from build123d import *

# Parameters (mm, degrees)
SKETCH1_W           = 8
SKETCH1_H           = 110
BOSS_EXTRUDE1_DEPTH = 40
SKETCH2_W           = 20
SKETCH2_H           = 24
CUT_EXTRUDE1_DEPTH  = 9
FILLET1_R           = 3
SKETCH3_R           = 1.25
CUT_EXTRUDE2_DEPTH  = 41


with BuildPart() as part:
    # Sketch1 → Boss-Extrude1 (new body)
    with BuildSketch(Plane.XY):
        Rectangle(SKETCH1_W, SKETCH1_H)
    extrude(amount=-BOSS_EXTRUDE1_DEPTH)

    # Sketch2 → Cut-Extrude1 (cut, through all)
    with BuildSketch(Plane(origin=(4, 0, 0), x_dir=(0, 0, -1), z_dir=(1, 0, 0))):
        with Locations((20, 55)):
            Rectangle(SKETCH2_W, SKETCH2_H)
        with Locations((20, -55)):
            Rectangle(SKETCH2_W, SKETCH2_H)
    extrude(amount=-CUT_EXTRUDE1_DEPTH, mode=Mode.SUBTRACT)

    # Fillet1
    fillet1_edges = [part.edges().sort_by_distance(p)[0] for p in [
        (4, 55, -5),
        (-4, 55, -5),
        (-4, -55, -5),
        (4, -55, -5),
        (4, -55, -35),
        (-4, -55, -35),
        (-4, 55, -35),
        (4, 55, -35),
    ]]
    fillet(fillet1_edges, radius=FILLET1_R)

    # Sketch3 → Cut-Extrude2 (cut, through all)
    with BuildSketch(Plane.XY):
        with Locations((0, 50)):
            Circle(SKETCH3_R)
        with Locations((0, -50)):
            Circle(SKETCH3_R)
    extrude(amount=-CUT_EXTRUDE2_DEPTH, mode=Mode.SUBTRACT)


solid = part.part
Part model, mm, in its own coordinate system. A direction names the side the tool comes from. Give positions to 0.01 mm unless a question says otherwise; leave off trailing zeros. Loops run counter-clockwise (first coordinate to the right, second up) from the corner with the lowest first, then second, coordinate; pieces in that order, holes last. Notation, with made-up numbers: (-29.5, -39) -> (-1.5, -39) arc R13 cw to (-1.5, -35) -> close; hole circle Ø8 at (5.5, 36.5). An arc over 180 degrees is marked (long way). Write each question's results on one line, items separated by ' | '. Start each with the question number.
Q1. Pin check, flat tips, straight feed: P1, Ø1.5, axis at x = 0, y = -50, coming from the +Z side; P2, Ø2.5, axis at x = -0.5, z = -15, coming from the +Y side; P3, Ø4, axis at x = -1, y = 47.5, coming from the +Z side. Stop position of each tip, or through.
Q2. Band-saw the part on A-A on y = 47. List the corners of the cut face in (x, z).
Q3. Band-saw the part on C-C on z = -33. List the corners of the cut face in (x, y), plus the area to 3 significant figures.
Q4. Pull direction Y, two halves, no side cores. Call faces 1 (the face through (-0.16, -48.76, -4.93)), 2 (the face through (0, -43, -20)), 3 (the face through (-4, -1, -20)): +Y half, -Y half, draft (parallel to the pull), parting line (faces both ways), or undercut.
Q5. Which spindle directions (+Z, -Z, +X, -X, +Y, -Y) get a long thin tool onto all of the face, cutting with end or side? Do faces 4 (the face through (1, 49, -30)), 5 (the face through (1, -49, -30)), 6 (the face through (0, -55, -5)). Say none if no direction does.
Q6. Band-saw the part on D-D on y = -50. List the corners of the cut face in (x, z), plus the area to 3 significant figures.
Q7. Wall check: L1, parallel to Y at x = 0, z = -35.5; L2, parallel to Y at x = -2, z = -11; L3, parallel to Y at x = -1.5, z = -31. Give the ranges that are in metal, low to high.
Q8. Band-saw the part on B-B on x = 0. List the corners of the cut face in (y, z), plus the area to 3 significant figures.
Results are:
1) P1: passes through | P2: stops at y = 43 | P3: stops at z = 0
2) outline: (-4, -40) -> (4, -40) -> (4, -30) -> (-4, -30) -> close; (-4, -10) -> (4, -10) -> (4, 0) -> (-4, 0) -> close
3) outline: (-4, -52) arc R3 ccw to (-1, -55) -> (1, -55) arc R3 ccw to (4, -52) -> (4, 52) arc R3 ccw to (1, 55) -> (-1, 55) arc R3 ccw to (-4, 52) -> close; hole circle Ø2.5 at (0, -50); hole circle Ø2.5 at (0, 50) | area: 862 mm²
4) face 1: undercut | face 2: -Y half | face 3: draft
5) face 4: +X, -X, +Y | face 5: +X, -X, -Y | face 6: +Z, -Z, +X, -X, -Y
6) outline: (-4, -40) -> (-1.25, -40) -> (-1.25, -30) -> (-4, -30) -> close; (-4, -10) -> (-1.25, -10) -> (-1.25, 0) -> (-4, 0) -> close; (1.25, -40) -> (4, -40) -> (4, -30) -> (1.25, -30) -> close; (1.25, -10) -> (4, -10) -> (4, 0) -> (1.25, 0) -> close | area: 110 mm²
7) L1: y = -55 to -51.25, -48.75 to 48.75, 51.25 to 55 | L2: y = -43 to 43 | L3: y = -54.96 to 54.96
8) outline: (-55, -40) -> (-51.25, -40) -> (-51.25, -30) -> (-55, -30) -> close; (-55, -10) -> (-51.25, -10) -> (-51.25, 0) -> (-55, 0) -> close; (-48.75, -40) -> (48.75, -40) -> (48.75, -30) -> (43, -30) -> (43, -10) -> (48.75, -10) -> (48.75, 0) -> (-48.75, 0) -> (-48.75, -10) -> (-43, -10) -> (-43, -30) -> (-48.75, -30) -> close; (51.25, -40) -> (55, -40) -> (55, -30) -> (51.25, -30) -> close; (51.25, -10) -> (55, -10) -> (55, 0) -> (51.25, 0) -> close | area: 3,820 mm²
